from build123d import *

# Parameters (mm, degrees)
F0_R      = 101.8057448426
F1_DEPTH  = 160
F2_R      = 28.5788941191
F3_DEPTH  = 120
F4_DEPTH  = 50
F6_W      = 90.1293829083
F6_H      = 44.228348881
F7_W      = 90.4394574463
F7_H      = 43.640833348
F8_DEPTH  = 76.2
F9_R      = 20.7879230701
F10_DEPTH = 101.6


with BuildPart() as f1:
    # F0 (on Top) → F1 (new body)
    with BuildSketch(Plane.XY):
        Circle(F0_R)
    extrude(amount=F1_DEPTH)

    # F2 (on face) → F3 (join)
    with BuildSketch(Plane.XY.offset(160)):
        Circle(F2_R)
    extrude(amount=F3_DEPTH)

    # F4 (add): a face of the model
    f4_faces = [f1.faces().sort_by_distance(p)[0] for p in [
        (0, 0, 0),
    ]]
    extrude(f4_faces, amount=F4_DEPTH)

    # F6 (on face) + F7 (on face) → F8 (join)
    with BuildSketch(Plane.XY.offset(280)):
        with Locations((-0.3652684391, -22.1141744405)):
            Rectangle(F6_W, F6_H)
    with BuildSketch(Plane.XY.offset(280)):
        with Locations((-1.5747603029, 21.820416674)):
            Rectangle(F7_W, F7_H)
    extrude(amount=F8_DEPTH)

    # F9 (on face) → F10 (join)
    with BuildSketch(Plane.XZ.offset(44.228348881)):
        with Locations((0, 322.1978545189)):
            Circle(F9_R)
    extrude(amount=F10_DEPTH)


solid = f1.part
Input: part model. Units: mm. Frame: model coordinates. A direction names the side the tool comes from. Give positions to 0.01 mm unless a question says otherwise; leave off trailing zeros. Loops run counter-clockwise (first coordinate to the right, second up) from the corner with the lowest first, then second, coordinate; pieces in that order, holes last. Notation, with made-up numbers: (23, 75.5) - (39, 75.5) arc R16 ccw to (39, 91.5) - close; hole circle Ø1 at (9.25, -17). An arc over 180 degrees is marked (long way). Use CSV: the item, a comma, the result in double quotes. Start each with the question number.
Item 1: Mould query, pull axis Z, two halves, no side actions, for faces 6 (the cylindrical face through (97.1, 30.6, 56.5)), 7 (the flat face through (-1, -44.228, 301)), 8 (the flat face through (-2, 0, 356.2)). Classes: pulls with the +Z half, pulls with the -Z half, needs draft (parallel to the pull), parting line crosses it, or undercut.
Item 2: Contact query for flat-ended pins moving along their axis: P1, Ø13.5, axis at y = -26, z = 330.5, coming from the +X side; P2, Ø4, axis at y = 16.5, z = 315.5, coming from the -X side; P3, Ø1.5, axis at y = 32, z = 82, coming from the +X side. Output: stop coordinate, or through.
Item 3: Reachability of faces 1 (the flat face through (44.699, -22, 318)), 2 (the cylindrical face through (9.592, -94.317, 303.755)), 3 (the flat face through (21, -21, 160)), 4 (the flat face through (43.645, 22, 318)), 5 (the flat face through (-2, 43.641, 318)) from +Z, -Z, +X, -X, +Y, -Y: full face, straight path, thin tool, end or side. Return the list, or none.
Item 4: Section A-A on x = 37. Return loops of the section in (y, z).
Item 5: Section D-D on x = 0. Return loops of the section in (y, z).
Item 6: Section B-B on y = -34.5. Return loops of the section in (x, z).
Item 7: Section C-C on z = 206. Return loops of the section in (x, y).
Item 8: Line query: line 1 (Z direction, x = -84.5, y = -1.5); line 2 (Y direction, x = -33.5, z = 325); line 3 (Z direction, x = 26.5, y = 22). Output: solid intervals per line, ascending.
Ans:
1,face 6,"needs draft"
1,face 7,"undercut"
1,face 8,"pulls with the +Z half"
2,P1,"stops at x = 44.7"
2,P2,"stops at x = -46.79"
2,P3,"stops at x = 96.89"
3,face 1,"+Z, +X, +Y, -Y"
3,face 2,"-Y"
3,face 3,"none"
3,face 4,"+Z, +X, +Y"
3,face 5,"+Z, +X, -X, +Y"
4,outline,"(-94.84, -50) - (94.84, -50) - (94.84, 160) - (-94.84, 160) - close; (-44.23, 280) - (43.64, 280) - (43.64, 356.2) - (-44.23, 356.2) - close"
5,outline,"(-145.83, 301.41) - (-44.23, 301.41) - (-44.23, 280) - (-28.58, 280) - (-28.58, 160) - (-101.81, 160) - (-101.81, -50) - (101.81, -50) - (101.81, 160) - (28.58, 160) - (28.58, 280) - (43.64, 280) - (43.64, 356.2) - (-44.23, 356.2) - (-44.23, 342.99) - (-145.83, 342.99) - close"
6,outline,"(-95.78, -50) - (95.78, -50) - (95.78, 160) - (-95.78, 160) - close; (-45.43, 280) - (44.7, 280) - (44.7, 356.2) - (-45.43, 356.2) - close"
7,outline,"circle Ø57.16 at (0, 0)"
8,line 1,"z = -50 to 160"
8,line 2,"y = -44.23 to 43.64"
8,line 3,"z = -50 to 160, 280 to 356.2"
